Check sheet for the modelled part. Datum: model origin and axes. Units: mm. Face numbers are marked on the shaded views. A direction names the side the tool comes from. Round coordinates to 2 decimals unless told otherwise and drop trailing zeros. Write each loop counter-clockwise with the first axis right and the second up, starting at its lowest first coordinate (ties: lowest second). Pieces come first, ordered by that corner, then holes. Notation, with made-up numbers: (-8.75, 58) -> (-3.75, 58) arc R17 cw to (-3.75, 87) -> close; hole circle Ø4 at (46.5, 74.5). An arc over 180 degrees is marked (long way). One line per item, written item: value.
from build123d import *

# Parameters (mm, degrees)
SKETCH_6_W          = 5
SKETCH_6_H          = 21
EXTRUDE_1_DEPTH     = 2
SKETCH_10_W         = 2
SKETCH_10_H         = 5
EXTRUDE_3_DEPTH     = 20
SKETCH_11_W         = 8
SKETCH_11_H         = 5
CUT_EXTRUDE_3_DEPTH = 20
SKETCH_12_R         = 1.5
CUT_EXTRUDE_4_DEPTH = 20
SKETCH_13_W         = 5
SKETCH_13_H         = 2
CUT_EXTRUDE_5_DEPTH = 8
FILLET_1_R          = 1.5
SKETCH_19_W         = 8
SKETCH_19_H         = 2
EXTRUDE_6_DEPTH     = 3
SKETCH_20_R         = 1.5
CUT_EXTRUDE_7_DEPTH = 5


with BuildPart() as part:
    # 草图6 → 凸台-拉伸1 (new body)
    with BuildSketch(Plane.XY):
        with Locations((-2.5, 10.5)):
            Rectangle(SKETCH_6_W, SKETCH_6_H)
    extrude(amount=EXTRUDE_1_DEPTH)

    # 草图10 → 凸台-拉伸3 (add)
    with BuildSketch(Plane(origin=(0, 0, 0), x_dir=(0, 0, -1), z_dir=(1, 0, 0))):
        with Locations((-1, 18.5)):
            Rectangle(SKETCH_10_W, SKETCH_10_H)
    extrude(amount=EXTRUDE_3_DEPTH)

    # 草图11 → 切除-拉伸3 (cut)
    with BuildSketch(Plane(origin=(0, 0, 0), x_dir=(-1, 0, 0), z_dir=(0, 0, -1))):
        with Locations((-16, 18.5)):
            Rectangle(SKETCH_11_W, SKETCH_11_H)
    extrude(amount=-CUT_EXTRUDE_3_DEPTH, mode=Mode.SUBTRACT)

    # 草图12 → 切除-拉伸4 (cut)
    with BuildSketch(Plane(origin=(0, 0, 0), x_dir=(-1, 0, 0), z_dir=(0, 0, -1))):
        with Locations((2.5, 18.5)):
            Circle(SKETCH_12_R)
    extrude(amount=-CUT_EXTRUDE_4_DEPTH, mode=Mode.SUBTRACT)

    # 草图13 → 切除-拉伸5 (cut)
    with BuildSketch(Plane.XZ):
        with Locations((-2.5, 1)):
            Rectangle(SKETCH_13_W, SKETCH_13_H)
    extrude(amount=-CUT_EXTRUDE_5_DEPTH, mode=Mode.SUBTRACT)

    # 圆角1
    fillet_1_edges = [part.edges().sort_by_distance(p)[0] for p in [
        (0, 8, 1),
        (-5, 8, 1),
    ]]
    fillet(fillet_1_edges, radius=FILLET_1_R)

    # 草图19 → 凸台-拉伸6 (add)
    with BuildSketch(Plane(origin=(0, 21, 0), x_dir=(1, 0, 0), z_dir=(0, 1, 0))):
        with Locations((-1, -1)):
            Rectangle(SKETCH_19_W, SKETCH_19_H)
    extrude(amount=EXTRUDE_6_DEPTH)

    # 草图20 → 切除-拉伸7 (cut)
    with BuildSketch(Plane(origin=(0, 0, 0), x_dir=(-1, 0, 0), z_dir=(0, 0, -1))):
        with Locations((-1, 21.5)):
            Circle(SKETCH_20_R)
    extrude(amount=-CUT_EXTRUDE_7_DEPTH, mode=Mode.SUBTRACT)


solid = part.part
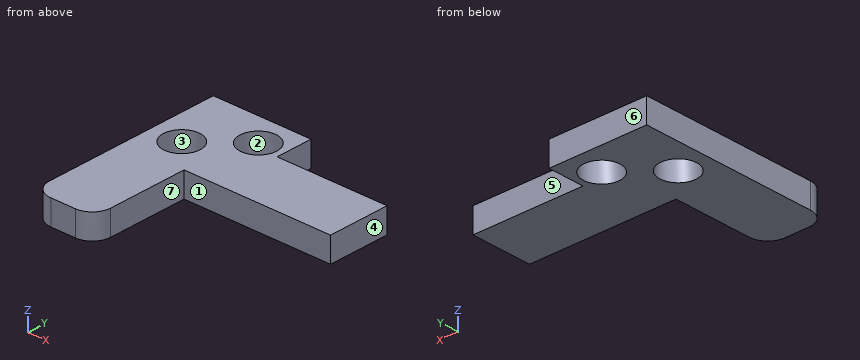
Item 1: Tool access check on the marked faces 5, 6 and 7. Record the directions out of +Z, -Z, +X, -X, +Y, -Y that give a thin tool (end or side, any length) a straight path to the whole face; none if there is none.
Answer:
face 5: +Z, -Z, +X, +Y
face 6: +Z, -Z, +X, -X, +Y
face 7: +Z, -Z, +X, -Y
Item 2: Sectioned sample at C-C on z = 1.6. Enter the section's corners in (x, y).
Answer:
outline: (-5, 9.5) arc R1.5 ccw to (-3.5, 8) -> (-1.5, 8) arc R1.5 ccw to (0, 9.5) -> (0, 16) -> (12, 16) -> (12, 21) -> (3, 21) -> (3, 24) -> (-5, 24) -> close; hole circle Ø3 at (-2.5, 18.5); hole circle Ø3 at (1, 21.5)
Item 3: Thickness scan on line 1 (Y direction, x = 1, z = 1.35); line 2 (X direction, y = 14, z = 1.2); line 3 (Y direction, x = -2.5, z = 0.6). Record the ranges inside material, lowest first.
Answer:
line 1: y = 16 to 20, 23 to 24
line 2: x = -5 to 0
line 3: y = 8 to 17, 20 to 24
Item 4: Depth check by flat-ended pin: P1, Ø1, axis at x = 6, z = 1, coming from the +Y side; P2, Ø1, axis at x = 3.5, z = 0.5, coming from the -Y side; P3, Ø1.8, axis at x = 1, y = 21.5, coming from the +Z side. Enter the tip coordinate at first touch or a pass-through.
Answer:
P1: stops at y = 21
P2: stops at y = 16
P3: passes through
Item 5: Sectioned sample at B-B on x = 1. Enter the section's corners in (y, z).
Answer:
outline: (16, 0) -> (20, 0) -> (20, 2) -> (16, 2) -> close; (23, 0) -> (24, 0) -> (24, 2) -> (23, 2) -> close
Item 6: Sectioned sample at A-A on y = 18.5. Enter the section's corners in (x, z).
Answer:
outline: (-5, 0) -> (-4, 0) -> (-4, 2) -> (-5, 2) -> close; (-1, 0) -> (12, 0) -> (12, 2) -> (-1, 2) -> close
Item 7: Mould release check, pull along Y, two halves, no side actions. Record for the marked faces 1, 2, 3 and 4: pulls with the +Y half, pulls with the -Y half, needs draft (parallel to the pull), parting line crosses it, or undercut.
Answer:
face 1: pulls with the -Y half
face 2: undercut
face 3: undercut
face 4: needs draft
Item 8: Sectioned sample at D-D on y = 10.5. Enter the section's corners in (x, z), and give its area (3 significant figures).
Answer:
outline: (-5, 0) -> (0, 0) -> (0, 2) -> (-5, 2) -> close
area: 10.0 mm^2
